Work out the finished part from the listing and answer in its coordinate system (mm). Give positions to 0.01 mm unless a question says otherwise; leave off trailing zeros. Write each loop counter-clockwise with the first axis right and the second up, starting at its lowest first coordinate (ties: lowest second). Pieces come first, ordered by that corner, then holes.
1) Straight lines are drawn through the part: probe 1 along Y at (x, z) = (52, 2.1); probe 2 along Y at (x, z) = (-120.5, 1.2); probe 3 along X at (y, z) = (-140, 2). For each, find the intervals that lie inside material, in ascending order.
2) Given pin 1 Ø1 at (y, z) = (-63.5, 2) entering from -X; pin 2 Ø0.9 at (x, z) = (89.5, 1.5) entering from -Y; pin 3 Ø0.9 at (x, z) = (98.5, 2) entering from +Y, each flat-ended and moving along its own axis, determine where each tip first touches the part or whether it passes through.
3) Find section A-A (z = 1.2). Count the separate pieces of the cut face and the enclosed holes in it, plus the area to 3 significant figures.
4) Find section B-B (y = 75.5). Determine the outline of the cut face in (x, z), plus the area to 3 significant figures.
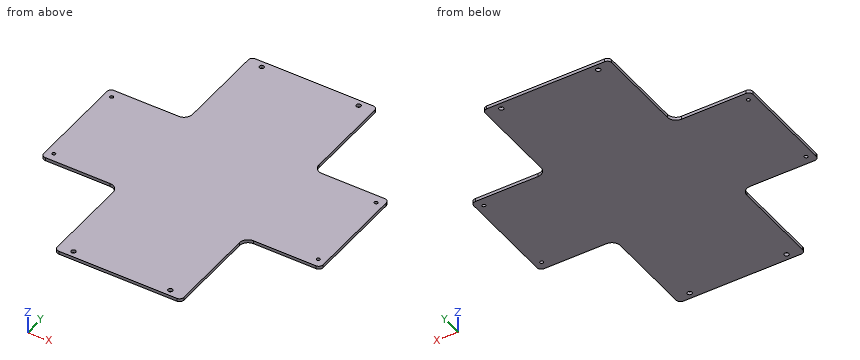
```python
from build123d import *

# Parameters (mm, degrees)
SKETCH_183_R   = 2.15
SKETCH_183_R_2 = 1.6
F_3MM_DEPTH    = 3


with BuildPart() as part:
    # Sketch 183 → 二层板_拉伸3mm (new body)
    with BuildSketch(Plane.XY):
        with BuildLine():
            Line((-50, -146), (62, -146))
            ThreePointArc((62, -146), (64.828427125, -144.828427125), (66, -142))
            Line((66, -142), (66, -59))
            ThreePointArc((66, -59), (68.343145751, -53.343145751), (74, -51))
            Line((74, -51), (133.5, -51))
            ThreePointArc((133.5, -51), (136.328427125, -49.828427125), (137.5, -47))
            Line((137.5, -47), (137.5, 47))
            ThreePointArc((137.5, 47), (136.328427125, 49.828427125), (133.5, 51))
            Line((133.5, 51), (74, 51))
            ThreePointArc((74, 51), (68.343145751, 53.343145751), (66, 59))
            Line((66, 59), (66, 142))
            ThreePointArc((66, 142), (64.828427125, 144.828427125), (62, 146))
            Line((62, 146), (-50, 146))
            ThreePointArc((-50, 146), (-52.828427125, 144.828427125), (-54, 142))
            Line((-54, 142), (-54, 59))
            ThreePointArc((-54, 59), (-56.343145751, 53.343145751), (-62, 51))
            Line((-62, 51), (-123.5, 51))
            ThreePointArc((-123.5, 51), (-126.328427125, 49.828427125), (-127.5, 47))
            Line((-127.5, 47), (-127.5, -47))
            ThreePointArc((-127.5, -47), (-126.328427125, -49.828427125), (-123.5, -51))
            Line((-123.5, -51), (-62, -51))
            ThreePointArc((-62, -51), (-56.343145751, -53.343145751), (-54, -59))
            Line((-54, -59), (-54, -142))
            ThreePointArc((-54, -142), (-52.828427125, -144.828427125), (-50, -146))
        make_face()
        with Locations((-40, 140)):
            Circle(SKETCH_183_R, mode=Mode.SUBTRACT)
        with Locations((52, 140)):
            Circle(SKETCH_183_R, mode=Mode.SUBTRACT)
        with Locations((-120.5, 43)):
            Circle(SKETCH_183_R_2, mode=Mode.SUBTRACT)
        with Locations((130.5, 43)):
            Circle(SKETCH_183_R_2, mode=Mode.SUBTRACT)
        with Locations((-120.5, -43)):
            Circle(SKETCH_183_R_2, mode=Mode.SUBTRACT)
        with Locations((130.5, -43)):
            Circle(SKETCH_183_R_2, mode=Mode.SUBTRACT)
        with Locations((-40, -140)):
            Circle(SKETCH_183_R, mode=Mode.SUBTRACT)
        with Locations((52, -140)):
            Circle(SKETCH_183_R, mode=Mode.SUBTRACT)
    extrude(amount=F_3MM_DEPTH)


solid = part.part
```
Results:
1. probe 1: y = -146 to -142.15, -137.85 to 137.85, 142.15 to 146
1. probe 2: y = -51 to -44.6, -41.4 to 41.4, 44.6 to 51
1. probe 3: x = -54 to -42.15, -37.85 to 49.85, 54.15 to 66
2. pin 1: stops at x = -54
2. pin 2: stops at y = -51
2. pin 3: stops at y = 51
3. separate pieces: 1
3. enclosed holes: 8
3. area: 49,800 mm2
4. outline: (-54, 0) - (66, 0) - (66, 3) - (-54, 3) - close
4. area: 360 mm2
